Verification items for this drawing (mm, ordinates from the low corner). A direction names the side the tool comes from. Round coordinates to 2 decimals unless told otherwise and drop trailing zeros. Loops run counter-clockwise (first coordinate to the right, second up) from the corner with the lowest first, then second, coordinate; pieces in that order, holes last. Notation, with made-up numbers: (3.5, 53) - (37.5, 53) arc R37 ccw to (37.5, 92) - close; hole circle Ø4 at (78.5, 49). An arc over 180 degrees is marked (long way). Put each result on its own line as item: value. Start each with the question number.
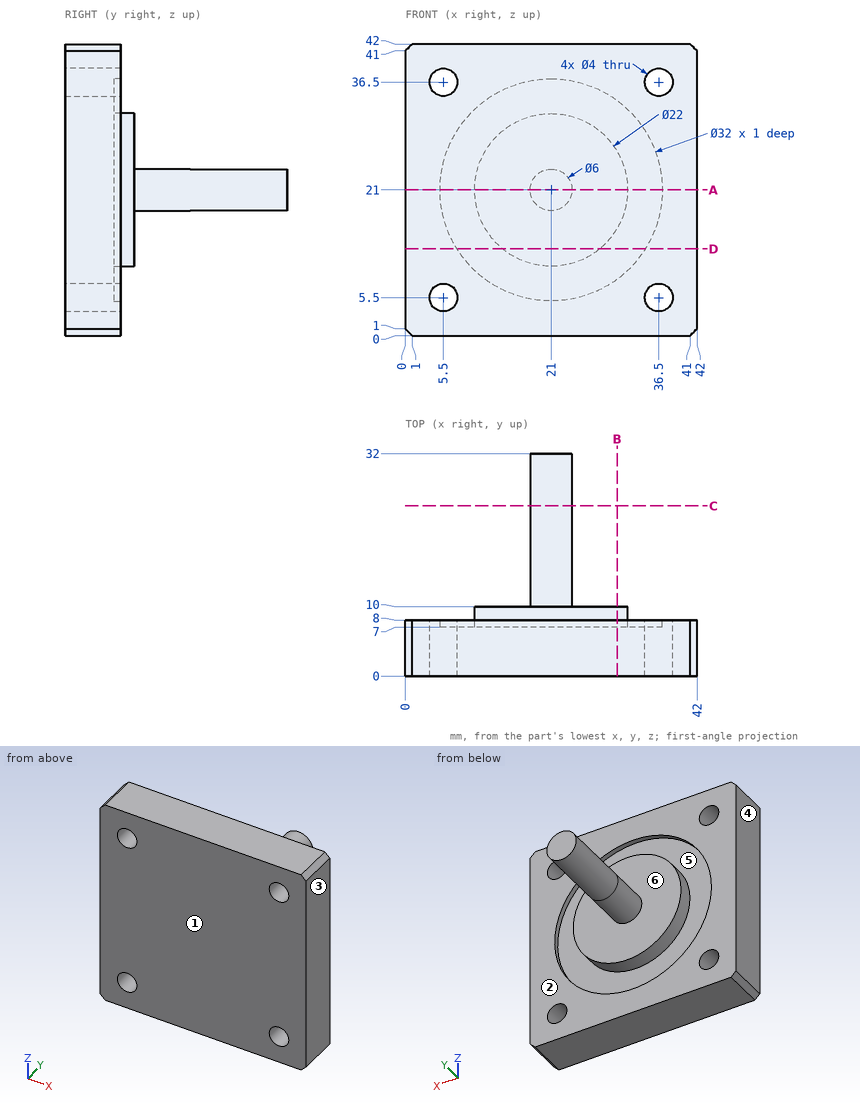
Q1. Cross-section at A-A on z = 21. Enter the section's corners in (x, y), and give its area (3 significant figures).
Q2. Draft check along X on the marked faces 3, 4, 5 and 6. Enter one of: +X half, -X half, draft (parallel to the pull), parting line (faces both ways), or undercut.
Q3. Set-up check for the marked faces 1 and 2: record each of +Z, -Z, +X, -X, +Y, -Y from which the full face is reachable in a straight line by a thin tool's end or side.
Q4. Cross-section at D-D on z = 12.5. Enter the section's corners in (x, y).
Q5. Material ranges on line 1 (X direction, y = 3.5, z = 36.5); line 2 (Y direction, x = 17.5, z = 29); line 3 (Y direction, x = 38, z = 38.5), recorded low to high. Write a range as from..to.
Q6. Cross-section at C-C on y = 24.5. Enter the section's corners in (x, z).
Q7. Cross-section at B-B on x = 30.5. Enter the section's corners in (y, z), and give its area (3 significant figures).
Q8. Depth check by flat-ended pin: pin 1 Ø12 at (y, z) = (24.5, 23.5) entering from -X; pin 2 Ø5 at (x, z) = (5.5, 36.5) entering from +Y; pin 3 Ø1 at (y, z) = (25.5, 22.5) entering from -X. Enter the tip coordinate at first touch or a pass-through.
Answer list:
1. outline: (0, 0) - (42, 0) - (42, 8) - (37, 8) - (37, 7) - (32, 7) - (32, 10) - (24, 10) - (24, 32) - (18, 32) - (18, 10) - (10, 10) - (10, 7) - (5, 7) - (5, 8) - (0, 8) - close
1. area: 502 mm2
2. face 3: +X half
2. face 4: -X half
2. face 5: undercut
2. face 6: draft
3. face 1: +Z, -Z, +X, -X, -Y
3. face 2: +Y
4. outline: (0, 0) - (42, 0) - (42, 8) - (34.56, 8) - (34.56, 7) - (27.98, 7) - (27.98, 10) - (14.02, 10) - (14.02, 7) - (7.44, 7) - (7.44, 8) - (0, 8) - close
5. line 1: x = 0..3.5, 7.5..34.5, 38.5..42
5. line 2: y = 0..10
5. line 3: y = 0..8
6. outline: circle Ø6 at (21, 21)
7. outline: (0, 0) - (8, 0) - (8, 8.13) - (7, 8.13) - (7, 15.45) - (10, 15.45) - (10, 26.55) - (7, 26.55) - (7, 33.87) - (8, 33.87) - (8, 42) - (0, 42) - close
7. area: 344 mm2
8. pin 1: stops at x = 18
8. pin 2: stops at y = 8
8. pin 3: stops at x = 18.17
